from build123d import *

# Parameters (mm, degrees)
SKETCH1_W = 32
SKETCH1_H = 4
SKETCH4_W = 0.94
SKETCH4_H = 1
SKETCH5_W = 0.94
SKETCH5_H = 1


with BuildPart() as part:
    # Sketch1 → Revolve1 (revolve)
    with BuildSketch(Plane.XY):
        with Locations((0, 2)):
            Rectangle(SKETCH1_W, SKETCH1_H)
    revolve(axis=Axis((16, 0, 0), (-1, 0, 0)))

    # Sketch2 → Cut-Revolve1 (revolve, cut)
    with BuildSketch(Plane.XY):
        Polygon((15, 4), (16, 3), (16, 4), align=None)
    revolve(axis=Axis((16, 0, 0), (-1, 0, 0)), mode=Mode.SUBTRACT)

    # Sketch3 → Cut-Revolve2 (revolve, cut)
    with BuildSketch(Plane.XY):
        Polygon((-16, 3), (-15, 4), (-16, 4), align=None)
    revolve(axis=Axis((16, 0, 0), (-1, 0, 0)), mode=Mode.SUBTRACT)

    # Sketch4 → Cut-Revolve3 (revolve, cut)
    with BuildSketch(Plane.XY):
        with Locations((12.97, 3.5)):
            Rectangle(SKETCH4_W, SKETCH4_H)
    revolve(axis=Axis((16, 0, 0), (-1, 0, 0)), mode=Mode.SUBTRACT)

    # Sketch5 → Cut-Revolve4 (revolve, cut)
    with BuildSketch(Plane.XY):
        with Locations((-12.97, 3.5)):
            Rectangle(SKETCH5_W, SKETCH5_H)
    revolve(axis=Axis((16, 0, 0), (-1, 0, 0)), mode=Mode.SUBTRACT)


solid = part.part
Here's how the part is built. I have some questions about the finished solid (model axes, mm). A direction names the side the tool comes from. Coordinates: 2 decimals unless noted, no trailing zeros. Write each loop counter-clockwise with the first axis right and the second up, starting at its lowest first coordinate (ties: lowest second). Pieces come first, ordered by that corner, then holes.
1) Which directions (+Z, -Z, +X, -X, +Y, -Y) give clear straight access to the entire face, cutting with the end or side of a thin tool? Please do faces 1 (the face through (13, -3, 0)), 2 (the face through (-14.209, -0.867, 3.905)).
Filled in:
face 1: none
face 2: +X, -X
2) If we section it at A-A (y = 0): List the corners of the cut face in (x, z) for me.
Filled in:
outline: (-16, -3) - (-15, -4) - (-13.44, -4) - (-13.44, -3) - (-12.5, -3) - (-12.5, -4) - (12.5, -4) - (12.5, -3) - (13.44, -3) - (13.44, -4) - (15, -4) - (16, -3) - (16, 3) - (15, 4) - (13.44, 4) - (13.44, 3) - (12.5, 3) - (12.5, 4) - (-12.5, 4) - (-12.5, 3) - (-13.44, 3) - (-13.44, 4) - (-15, 4) - (-16, 3) - close
3) If we section it at D-D (z = 3.5): Count the separate pieces of the cut face and the enclosed holes in it, plus the area to 3 significant figures.
Filled in:
separate pieces: 3
enclosed holes: 0
area: 111 mm2
4) If we section it at C-C (x = -4.5): List the corners of the cut face in (y, z) for me, plus the area to 3 significant figures.
Filled in:
outline: circle Ø8 at (0, 0)
area: 50.3 mm2
5) I'm going to push flat-ended pins straight in: pin 1 (3 mm diameter, centred on x = -6, y = -2, fed in from -Z); pin 2 (1.5 mm diameter, centred on x = 11, y = -2.5, fed in from +Z). Where does each tip first touch, or does it pass through?
Filled in:
pin 1: stops at z = -3.97
pin 2: stops at z = 3.6
6) If I drill on line 1 (X direction, y = 1.5, z = -2.75); line 2 (X direction, y = 3.5, z = -1.5); line 3 (Y direction, x = 11, z = 1.75), over which ranges is the centre line in solid material (lowest first)?
Filled in:
line 1: x = -15.87 to -13.44, -12.5 to 12.5, 13.44 to 15.87
line 2: x = -15.19 to -13.44, -12.5 to 12.5, 13.44 to 15.19
line 3: y = -3.6 to 3.6
7) Thinking about a two-plate mould opening in X: for faces 3 (the face through (16, 0, 0)), 4 (the face through (-16, 0, 0)), 5 (the face through (14.231, -0.867, 3.905)), 6 (the face through (-13.44, -1, -3)), which applies, +X half, -X half, draft (parallel to the pull), parting line (faces both ways), or undercut?
Filled in:
face 3: +X half
face 4: -X half
face 5: draft
face 6: undercut
